```python
from build123d import *

# Parameters (mm, degrees)
SKETCH_1_R      = 1.6
SKETCH_1_R_2    = 0.95
EXTRUDE_1_DEPTH = 3


with BuildPart() as part:
    # 草图1 → 凸台-拉伸1 (new body)
    with BuildSketch(Plane.XY):
        with BuildLine():
            Line((32, 23.279914581), (63, 23.279914581))
            ThreePointArc((63, 23.279914581), (64.664100589, 22.776065464), (65.769230769, 21.433760735))
            Line((65.769230769, 21.433760735), (66.730769231, 19.126068427))
            Line((66.730769231, 19.126068427), (69.29930559, 12.961581165))
            ThreePointArc((69.29930559, 12.961581165), (70.404435771, 11.619276436), (72.068536359, 11.115427319))
            Line((72.068536359, 11.115427319), (99.5, 11.115427319))
            ThreePointArc((99.5, 11.115427319), (101.621320344, 11.994106975), (102.5, 14.115427319))
            Line((102.5, 14.115427319), (102.5, 78.115427319))
            ThreePointArc((102.5, 78.115427319), (101.621320344, 80.236747662), (99.5, 81.115427319))
            Line((99.5, 81.115427319), (-4.5, 81.115427319))
            ThreePointArc((-4.5, 81.115427319), (-6.621320344, 80.236747662), (-7.5, 78.115427319))
            Line((-7.5, 78.115427319), (-7.5, 14.115427319))
            ThreePointArc((-7.5, 14.115427319), (-6.621320344, 11.994106975), (-4.5, 11.115427319))
            Line((-4.5, 11.115427319), (22.931463641, 11.115427319))
            ThreePointArc((22.931463641, 11.115427319), (24.595564229, 11.619276436), (25.70069441, 12.961581165))
            Line((25.70069441, 12.961581165), (28.269230769, 19.126068427))
            Line((28.269230769, 19.126068427), (29.230769231, 21.433760735))
            ThreePointArc((29.230769231, 21.433760735), (30.335899411, 22.776065464), (32, 23.279914581))
        make_face()
        with Locations((0, 34.5)):
            Circle(SKETCH_1_R, mode=Mode.SUBTRACT)
        with Locations((0, 27)):
            Circle(SKETCH_1_R, mode=Mode.SUBTRACT)
        with Locations((95, 34.5)):
            Circle(SKETCH_1_R, mode=Mode.SUBTRACT)
        with Locations((95, 27.1)):
            Circle(SKETCH_1_R, mode=Mode.SUBTRACT)
        with Locations((13.75, 76.079914581)):
            Circle(SKETCH_1_R_2, mode=Mode.SUBTRACT)
        with Locations((81.25, 76.079914581)):
            Circle(SKETCH_1_R_2, mode=Mode.SUBTRACT)
        with Locations((69.5, 20.079914581)):
            Circle(SKETCH_1_R_2, mode=Mode.SUBTRACT)
        with Locations((25.5, 20.079914581)):
            Circle(SKETCH_1_R_2, mode=Mode.SUBTRACT)
    extrude(amount=EXTRUDE_1_DEPTH)


solid = part.part
```
Build history of the part. All positions in model axes, mm. A direction names the side the tool comes from. Round coordinates to 2 decimals unless told otherwise and drop trailing zeros. Loops run counter-clockwise (first coordinate to the right, second up) from the corner with the lowest first, then second, coordinate; pieces in that order, holes last.
Item 1: Saw through at A-A (y = 34.5). List the corners of the cut face in (x, z).
Item 2: Saw through at C-C (z = 1.4). State how many separate pieces and enclosed holes the cut face has, then the cut area to 3 significant figures.
Item 3: Which spindle directions (+Z, -Z, +X, -X, +Y, -Y) get a long thin tool onto all of the face, cutting with end or side? Do faces 1 (the face through (47, 23.28, 1)), 2 (the face through (-7.5, 47, 1)). Say none if no direction does.
Item 4: Pin check, flat tips, straight feed: P1, Ø4, axis at x = 0, y = 27, coming from the +Z side; P2, Ø2.5, axis at x = 0, y = 34.5, coming from the -Z side; P3, Ø1.5, axis at x = 43.5, z = 2, coming from the -Y side. Stop position of each tip, or through.
Item 5: Two-plate mould, pull along X, no slides. Class faces 3 (the face through (-6.645, 12.018, 1.479)), 4 (the face through (93.4, 34.57, 1.48)), 5 (the face through (70.384, 11.633, 1.479)), 6 (the face through (86, 11.115, 1)): released by +X, released by -X, zero draft, split by the parting line, or undercut.
Item 6: Saw through at D-D (x = 41.5). List the corners of the cut face in (y, z).
Item 7: Saw through at B-B (x = 0). List the corners of the cut face in (y, z), then the cut area to 3 significant figures.
Item 8: Drill centre lines: line 1 along Y through (x, z) = (95, 1.8); line 2 along Y through (x, z) = (81.25, 2.05); line 3 along X through (y, z) = (22.5, 1.85). Where is each one in solid material? Low to high.
Worked answers:
1. outline: (-7.5, 0) - (-1.6, 0) - (-1.6, 3) - (-7.5, 3) - close; (1.6, 0) - (93.4, 0) - (93.4, 3) - (1.6, 3) - close; (96.6, 0) - (102.5, 0) - (102.5, 3) - (96.6, 3) - close
2. separate pieces: 1
2. enclosed holes: 8
2. area: 7,160 mm2
3. face 1: +Z, -Z, -Y
3. face 2: +Z, -Z, -X, +Y, -Y
4. P1: stops at z = 3
4. P2: passes through
4. P3: stops at y = 23.28
5. face 3: released by -X
5. face 4: undercut
5. face 5: undercut
5. face 6: zero draft
6. outline: (23.28, 0) - (81.12, 0) - (81.12, 3) - (23.28, 3) - close
7. outline: (11.12, 0) - (25.4, 0) - (25.4, 3) - (11.12, 3) - close; (28.6, 0) - (32.9, 0) - (32.9, 3) - (28.6, 3) - close; (36.1, 0) - (81.12, 0) - (81.12, 3) - (36.1, 3) - close
7. area: 191 mm2
8. line 1: y = 11.12 to 25.5, 28.7 to 32.9, 36.1 to 81.12
8. line 2: y = 11.12 to 75.13, 77.03 to 81.12
8. line 3: x = -7.5 to 29.98, 65.02 to 102.5
